```python
from build123d import *

# Parameters (mm, degrees)
SKETCH1_W           = 196.85
SKETCH1_H           = 200.025
BOSS_EXTRUDE1_DEPTH = 5.9944
SKETCH2_R           = 1.778
SKETCH2_R_2         = 1.35255
SKETCH2_W           = 5.9944
SKETCH2_H           = 25.4
SKETCH2_W_2         = 6.35
SKETCH2_H_2         = 5.9944
CUT_EXTRUDE1_DEPTH  = 6.9944
SKETCH3_W           = 5.9944
SKETCH3_H           = 3.175
BOSS_EXTRUDE2_DEPTH = 5.9944


with BuildPart() as part:
    # Sketch1 → Boss-Extrude1 (new body)
    with BuildSketch(Plane.XY):
        with Locations((98.425, 100.0125)):
            Rectangle(SKETCH1_W, SKETCH1_H)
    extrude(amount=-BOSS_EXTRUDE1_DEPTH)

    # Sketch2 → Cut-Extrude1 (cut, through all)
    with BuildSketch(Plane.XY):
        with Locations((191.77, 193.675)):
            Circle(SKETCH2_R)
        with Locations((191.77, 100.0125)):
            Circle(SKETCH2_R)
        with Locations((191.77, 6.35)):
            Circle(SKETCH2_R)
        with Locations((3.175, 3.175)):
            Circle(SKETCH2_R_2)
        with Locations((6.1722, 174.625)):
            Circle(SKETCH2_R)
        with Locations((6.1722, 19.05)):
            Circle(SKETCH2_R)
        with Locations((191.77, 158.75)):
            Rectangle(SKETCH2_W, SKETCH2_H)
        with Locations((191.77, 41.275)):
            Rectangle(SKETCH2_W, SKETCH2_H)
        Polygon((7.9248, 189.103), (7.9248, 191.2874), (10.9728, 191.2874), (10.9728, 189.103), (15.875, 189.103), (15.875, 185.547), (10.9728, 185.547), (10.9728, 183.3626), (7.9248, 183.3626), (7.9248, 185.547), (0, 185.547), (0, 189.103), align=None)
        with Locations((9.525, 2.9972)):
            Rectangle(SKETCH2_W_2, SKETCH2_H_2)
    extrude(amount=-CUT_EXTRUDE1_DEPTH, mode=Mode.SUBTRACT)

    # Sketch3 → Boss-Extrude2 (add)
    with BuildSketch(Plane.XY):
        with Locations((-2.9972, 198.4375)):
            Rectangle(SKETCH3_W, SKETCH3_H)
        with Locations((-2.9972, 176.2125)):
            Rectangle(SKETCH3_W, SKETCH3_H)
    extrude(amount=-BOSS_EXTRUDE2_DEPTH)


solid = part.part
```
Source: CAD feature listing. Evaluate the final solid. Frame: model axes, mm. A direction names the side the tool comes from. Round coordinates to 2 decimals unless told otherwise and drop trailing zeros. Loops run counter-clockwise (first coordinate to the right, second up) from the corner with the lowest first, then second, coordinate; pieces in that order, holes last.
(1) Pull-direction query (X, two-part tool) for faces 1 (the flat face through (192, 28.575, -3)), 2 (the flat face through (192, 53.975, -3)), 3 (the flat face through (0, 193, -3)), 4 (the flat face through (-3, 174.625, -3)); classes: +X half, -X half, draft (parallel to the pull), parting line (faces both ways), or undercut.
From the geometry:
face 1: undercut
face 2: undercut
face 3: -X half
face 4: draft
(2) Access query for faces 5 (the flat face through (13, 185.547, -3)), 6 (the flat face through (9, 5.994, -3)), 7 (the flat face through (196.85, 99, -3)), 8 (the flat face through (94, 101, 0)), 9 (the flat face through (188.773, 159, -3)). Directions: +Z, -Z, +X, -X, +Y, -Y. A direction counts if a zero-diameter tool reaches every point of the face in a straight line with its end or side. Return the directions, or none.
From the geometry:
face 5: +Z, -Z, -X
face 6: +Z, -Z, -Y
face 7: +Z, -Z, +X, +Y, -Y
face 8: +Z, +X, -X, +Y, -Y
face 9: +Z, -Z
(3) Material intervals for probe 1 along X at (y, z) = (157.5, -2.6); probe 2 along X at (y, z) = (56, -3.9); probe 3 along X at (y, z) = (18, -4.4), sorted ascending.
From the geometry:
probe 1: x = 0 to 188.77, 194.77 to 196.85
probe 2: x = 0 to 196.85
probe 3: x = 0 to 4.74, 7.61 to 196.85
(4) Section query A-A (y = 159.5). Output: boundary loops of the cut face in (x, z).
From the geometry:
outline: (0, -5.99) - (188.77, -5.99) - (188.77, 0) - (0, 0) - close; (194.77, -5.99) - (196.85, -5.99) - (196.85, 0) - (194.77, 0) - close
(5) Contact query for flat-ended pins moving along their axis: pin 1 Ø3 at (y, z) = (66, -4) entering from -X; pin 2 Ø3 at (x, z) = (-3.5, -4.5) entering from -Y (3 decimals); pin 3 Ø2.5 at (x, z) = (9.5, -3) entering from -Y. Output: stop coordinate, or through.
From the geometry:
pin 1: stops at x = 0
pin 2: stops at y = 174.625
pin 3: stops at y = 5.99
(6) Section query B-B (z = -4.15). Give the number of separate pieces and of enclosed holes in the cut face, and give its area (3 significant figures).
From the geometry:
separate pieces: 1
enclosed holes: 8
area: 38,900 mm2
